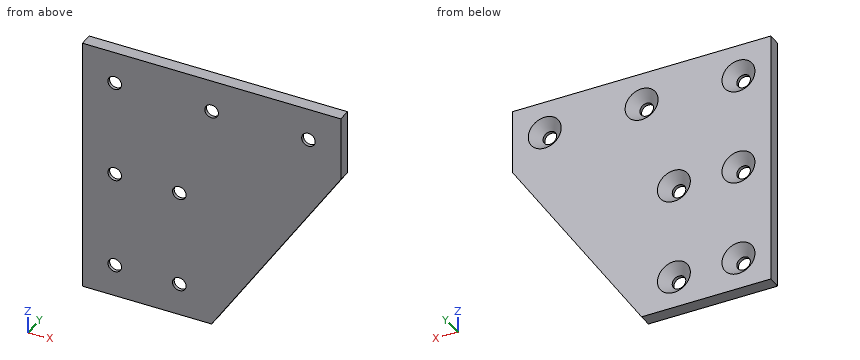
from build123d import *

# Parameters (mm, degrees)
BOSS_EXTRUDE1_DEPTH = 4
SKETCH2_R           = 2.1
CUT_EXTRUDE1_DEPTH  = 4
CHAMFER1_SIZE       = 3


with BuildPart() as part:
    # Sketch1 → Boss-Extrude1 (new body)
    with BuildSketch(Plane(origin=(0, 0, 0), x_dir=(1, 0, 0), z_dir=(0, 1, 0))):
        Polygon((0, 0), (80, 0), (80, 20), (40, 80), (0, 80), align=None)
    extrude(amount=BOSS_EXTRUDE1_DEPTH)

    # Sketch2 → Cut-Extrude1 (cut)
    with BuildSketch(Plane(origin=(0, 4, 0), x_dir=(1, 0, 0), z_dir=(0, 1, 0))):
        with Locations((10, 10)):
            Circle(SKETCH2_R)
        with Locations((40, 10)):
            Circle(SKETCH2_R)
        with Locations((70, 10)):
            Circle(SKETCH2_R)
        with Locations((30, 40)):
            Circle(SKETCH2_R)
        with Locations((30, 70)):
            Circle(SKETCH2_R)
        with Locations((10, 40)):
            Circle(SKETCH2_R)
        with Locations((10, 70)):
            Circle(SKETCH2_R)
    extrude(amount=-CUT_EXTRUDE1_DEPTH, mode=Mode.SUBTRACT)

    # Chamfer1
    chamfer1_edges = [part.edges().sort_by_distance(p)[0] for p in [
        (7.9, 4, -70),
        (7.9, 4, -40),
        (27.9, 4, -70),
        (27.9, 4, -40),
        (67.9, 4, -10),
        (37.9, 4, -10),
        (7.9, 4, -10),
    ]]
    chamfer(chamfer1_edges, length=CHAMFER1_SIZE)


solid = part.part
The listing builds one solid part. Answer for the finished solid, in the listing's coordinates (mm). Coordinates: 2 decimals unless noted, no trailing zeros. Loops run counter-clockwise (first coordinate to the right, second up) from the corner with the lowest first, then second, coordinate; pieces in that order, holes last.
1) Find the intervals of material crossed by L1, parallel to Z at x = 10, y = 0.4; L2, parallel to Z at x = 30, y = 0.6; L3, parallel to X at y = 0.7, z = -10, in increasing order.
2) Find section C-C on z = -10. Write down the section's boundary in (x, y), then the cut area to 3 significant figures.
3) Flat-ended cylindrical pins translate along their axes: pin 1 Ø4 at (x, z) = (30, -40) entering from -Y; pin 2 Ø6 at (x, z) = (69.5, -35.5) entering from -Y; pin 3 Ø5 at (x, z) = (10, -70) entering from +Y; pin 4 Ø5.5 at (x, z) = (30, -70) entering from +Y. Find the tip coordinate at first contact, or state that the pin passes through.
4) Find section D-D on x = 30. Write down the section's boundary in (y, z).
5) Find section B-B on y = 3.15. Write down the section's boundary in (x, z), then the cut area to 3 significant figures.
6) Find section A-A on x = 10. Write down the section's boundary in (y, z).
Values:
1. L1: z = -80 to -72.1, -67.9 to -42.1, -37.9 to -12.1, -7.9 to 0
1. L2: z = -80 to -72.1, -67.9 to -42.1, -37.9 to 0
1. L3: x = 0 to 7.9, 12.1 to 37.9, 42.1 to 67.9, 72.1 to 80
2. outline: (0, 0) - (7.9, 0) - (7.9, 1) - (4.9, 4) - (0, 4) - close; (12.1, 0) - (37.9, 0) - (37.9, 1) - (34.9, 4) - (15.1, 4) - (12.1, 1) - close; (42.1, 0) - (67.9, 0) - (67.9, 1) - (64.9, 4) - (45.1, 4) - (42.1, 1) - close; (72.1, 0) - (80, 0) - (80, 4) - (75.1, 4) - (72.1, 1) - close
2. area: 243 mm2
3. pin 1: passes through
3. pin 2: stops at y = 0
3. pin 3: stops at y = 1.4
3. pin 4: stops at y = 1.65
4. outline: (0, -80) - (4, -80) - (4, -75.1) - (1, -72.1) - (0, -72.1) - close; (0, -67.9) - (1, -67.9) - (4, -64.9) - (4, -45.1) - (1, -42.1) - (0, -42.1) - close; (0, -37.9) - (1, -37.9) - (4, -34.9) - (4, 0) - (0, 0) - close
5. outline: (0, -80) - (40, -80) - (80, -20) - (80, 0) - (0, 0) - close; hole circle Ø8.5 at (10, -70); hole circle Ø8.5 at (10, -40); hole circle Ø8.5 at (10, -10); hole circle Ø8.5 at (30, -70); hole circle Ø8.5 at (30, -40); hole circle Ø8.5 at (40, -10); hole circle Ø8.5 at (70, -10)
5. area: 4,800 mm2
6. outline: (0, -80) - (4, -80) - (4, -75.1) - (1, -72.1) - (0, -72.1) - close; (0, -67.9) - (1, -67.9) - (4, -64.9) - (4, -45.1) - (1, -42.1) - (0, -42.1) - close; (0, -37.9) - (1, -37.9) - (4, -34.9) - (4, -15.1) - (1, -12.1) - (0, -12.1) - close; (0, -7.9) - (1, -7.9) - (4, -4.9) - (4, 0) - (0, 0) - close
